Verification items for the finished model (mm, model axes). A direction names the side the tool comes from. Give positions to 0.01 mm unless a question says otherwise; leave off trailing zeros. Loops run counter-clockwise (first coordinate to the right, second up) from the corner with the lowest first, then second, coordinate; pieces in that order, holes last. Notation, with made-up numbers: (41.5, 34.5) - (58.5, 34.5) arc R12 cw to (58.5, 38.5) - close; hole circle Ø10 at (-20.5, 62). An arc over 180 degrees is marked (long way). One line per question, with ' | ' between items. Start each with the question number.
1. Section check D-D, the plane x = 56. Enter the section's corners in (y, z) (3 decimals).
2. Mould release check, pull along Z, two halves, no side actions. Record for faces 1 (the face through (76.09, 1.61, -137.79)), 2 (the face through (47, 3.175, -100)), 3 (the face through (1.91, 1.57, -71.66)), 4 (the face through (123.55, 1.57, -38.69)): +Z half, -Z half, draft (parallel to the pull), parting line (faces both ways), or undercut.
3. Tool access check on faces 5 (the face through (106.04, 1.57, -106.59)), 6 (the face through (128, 2, -126)). Record the directions out of +Z, -Z, +X, -X, +Y, -Y that give a thin tool (end or side, any length) a straight path to the whole face; none if there is none.
4. Depth check by flat-ended pin: pin 1 Ø17 at (x, z) = (135.68, -58.14) entering from -Y. Enter the tip coordinate at first touch or a pass-through.
5. Section check A-A, the plane z = -64. Enter the section's corners in (x, y) (3 decimals), then the cut area to 3 significant figures.
6. Section check C-C, the plane y = 0.95. State how many separate pieces and enclosed holes the cut face has, then the cut area to 3 significant figures.
7. Section check B-B, the plane x = 95. Enter the section's corners in (y, z) (3 decimals).
8. Thickness scan on line 1 along X through (y, z) = (0.85, -35.5); line 2 along Z through (x, y) = (157, 0.7); line 3 along X through (y, z) = (2.1, -85.5). Record the ranges inside material, lowest first. Write a range as from..to.
Autodesk Inventor part; units mm, degrees
ref_plane "YZ Plane" through (0, 0, 0) normal (1, 0, 0) x (0, 1, 0)
ref_plane "XZ Plane" through (0, 0, 0) normal (0, 1, 0) x (-1, 0, 0)
ref_plane "XY Plane" through (0, 0, 0) normal (0, 0, 1) x (1, 0, 0)
sketch "Sketch1" plane through (0, 0, 0) normal (0, 1, 0) x (-1, 0, 0)
  line L0 (0, 0) -> (-165.1, 0)
  line L1 (-165.1, 0) -> (-165.1, -165.1)
  line L2 (-165.1, -165.1) -> (0, -165.1)
  line L3 (0, -165.1) -> (0, 0)
  circle A0 centre (-79.375, -79.375) radius 38.1
  line L4 (-25.4, -165.1) -> (-25.4, 0) construction
  line L5 (0, -25.4) -> (-165.1, -25.4) construction
  line L6 (0, 0) -> (-165.1, -165.1) construction
  circle A1 centre (-79.375, -79.375) radius 53.975 construction
  dimension "d0" = 76.2
  dimension "d3" = 25.4
  dimension "d4" = 25.4
  dimension "d5" = 107.95
  dimension "d25" = 165.1
extrude "Extrusion1" add sketch "Sketch1" along normal blind 3.175
sketch "Sketch2" plane through (0, 3.175, 0) normal (0, 1, 0) x (1, 0, 0)
  circle A0 centre (79.375, 79.375) radius 38.1 construction
  circle A1 centre (79.375, 79.375) radius 60.325 construction
  line L0 (0, 165.1) -> (0, 0) construction
  arc A2 (184.15, 82.55) -> (82.55, 184.15) centre (82.55, 82.55) ccw construction
  line L1 (36.7188, 36.7188) -> (122.0312, 36.7188) construction
  line L2 (122.0312, 36.7188) -> (122.0312, 122.0312) construction
  line L3 (122.0312, 122.0312) -> (36.7188, 122.0312) construction
  line L4 (36.7188, 122.0312) -> (36.7188, 36.7188) construction
  dimension "d9" = 120.65
hole "Hole1" at (36.7188, 3.175, -36.7188) at (122.0312, 3.175, -122.0312) at (122.0312, 3.175, -36.7188) at (36.7188, 3.175, -122.0312) direction (0, -1, 0) diameter 4.9784 end through all
sketch "Sketch3" plane through (0, 3.175, 0) normal (0, 1, 0) x (1, 0, 0)
  circle A0 centre (79.375, 79.375) radius 38.1 construction
  circle A1 centre (79.375, 79.375) radius 53.975 construction
  circle A2 centre (58.1423, 135.6764) radius 9.525
  line L0 (0, 0) -> (79.375, 79.375) construction
  circle A3 centre (135.6764, 58.1423) radius 9.525
  circle A4 centre (122.0312, 122.0312) radius 2.4892 construction
  circle A5 centre (58.1423, 135.6764) radius 24.13 construction
  line L1 (79.375, 79.375) -> (78.4947, 148.6394) construction
  circle A6 centre (78.4947, 148.6394) radius 11.1125
  circle A7 centre (148.6394, 78.4947) radius 11.1125
  circle A8 centre (58.1423, 135.6764) radius 25.4 construction
  circle A9 centre (122.0312, 122.0312) radius 4.7625 construction
  circle A10 centre (58.1423, 135.6764) radius 29.9974 construction
  circle A11 centre (36.7188, 122.0312) radius 2.4892
  circle A12 centre (44.4971, 157.1) radius 2.4892
  circle A13 centre (122.0312, 36.7188) radius 2.4892
  circle A14 centre (157.1, 44.4971) radius 2.4892
  circle A15 centre (71.7875, 114.2529) radius 2.4892
  circle A16 centre (114.2529, 71.7875) radius 2.4892
  circle A17 centre (79.375, 79.375) radius 38.1
  arc A18 (52.3602, 106.2416) -> (81.9214, 117.3898) centre (58.1423, 135.6764) ccw
  arc A19 (117.3898, 81.9214) -> (106.2416, 52.3602) centre (135.6764, 58.1423) ccw
  circle A20 centre (36.7188, 122.0312) radius 2.4892
  line L2 (36.7188, 122.0312) -> (78.4947, 148.6394) construction
  point P0 (117.3898, 81.9214)
  point P1 (106.2416, 52.3602)
  dimension "d33" = 48.26
  dimension "d17" = 107.95
  dimension "d19" = 19.05
  dimension "d34" = 69.27
  dimension "d35" = 22.225
  dimension "d37" = 50.8
  dimension "d38" = 59.9948
  dimension "d39" = 9.525
  dimension "d52" = 4.9784
  dimension "d53" = 90
  dimension "d56" = 90
extrude "Extrusion5" cut sketch "Sketch3" against normal through all contours A2 | A3 | A6 | A7 | A12 | A14 | A15 A17 | A17 A15 | A17 A16 | A16 A17
extrude "Extrusion6" add sketch "Sketch3" against normal up to surface (3.175 mm away) contours A15 A17 A18 | A17 A16 A19
sketch "Sketch5" plane through (0, 3.175, 0) normal (0, 1, 0) x (1, 0, 0)
  line L0 (0, 165.1) -> (0, 0)
  line L1 (0, 0) -> (25.4, 0)
  line L2 (25.4, 0) -> (25.4, 69.85)
  line L3 (25.4, 69.85) -> (0, 69.85)
  line L4 (0, 69.85) -> (0, 0)
  line L5 (25.4, 0) -> (69.85, 0)
  line L6 (69.85, 0) -> (69.85, 25.4)
  line L7 (69.85, 25.4) -> (25.4, 25.4)
  line L8 (25.4, 25.4) -> (25.4, 0)
  dimension "d63" = 25.4
  dimension "d64" = 69.85
  dimension "d65" = 44.45
  dimension "d66" = 25.4
extrude "Extrusion7" cut sketch "Sketch5" against normal up to surface (3.175 mm away)
chamfer "Chamfer3" distance 76.2 angle 45 1 edges at (165.1, 1.5875, -165.1)
fillet "Fillet6" radius 6.35 7 edges at (165.1, 1.5875, 0) (165.1, 1.5875, -88.9) (88.9, 1.5875, -165.1) (0, 1.5875, -165.1) (25.4, 1.5875, -25.4) (0, 1.5875, -69.85) (69.85, 1.5875, 0)
properties part number "TopPlate2"
Results list:
1) outline: (0, -165.1) - (3.175, -165.1) - (3.175, -144.957) - (0, -144.957) - close; (0, -126.395) - (3.175, -126.395) - (3.175, -105.756) - (0, -105.756) - close; (0, -49.288) - (3.175, -49.288) - (3.175, -25.4) - (0, -25.4) - close
2) face 1: undercut | face 2: draft | face 3: +Z half | face 4: undercut
3) face 5: +Y, -Y | face 6: -Z, +X, +Y, -Y
4) pin 1: through
5) outline: (25.4, 0) - (44.515, 0) - (44.515, 3.175) - (25.4, 3.175) - close; (106.256, 0) - (128.166, 0) - (128.166, 3.175) - (106.256, 3.175) - close; (143.187, 0) - (165.1, 0) - (165.1, 3.175) - (143.187, 3.175) - close | area: 200 mm²
6) separate pieces: 1 | enclosed holes: 13 | area: 15,700 mm²
7) outline: (0, -159) - (3.175, -159) - (3.175, -114.124) - (0, -114.124) - close; (0, -44.626) - (3.175, -44.626) - (3.175, 0) - (0, 0) - close
8) line 1: 25.4..34.55, 38.89..119.86, 124.2..165.1 | line 2: -97..-85.82, -71.17..-46.98, -42.01..0 | line 3: 0..41.77, 116.98..140.01, 157.27..165.1
